Verification items for the finished model (mm, model axes). A direction names the side the tool comes from. Round coordinates to 2 decimals unless told otherwise and drop trailing zeros. Write each loop counter-clockwise with the first axis right and the second up, starting at its lowest first coordinate (ties: lowest second). Pieces come first, ordered by that corner, then holes. Notation, with made-up numbers: M 81.25,-1.75 L 89.25,-1.75 A36 cw 89.25,35.25 Z; hole C 3,-17 d4. An arc over 180 degrees is marked long. One line per question, with ' | ' between items.
from build123d import *

# Parameters (mm, degrees)
F0_W     = 278.8
F0_H     = 12.5
F4_DEPTH = 4
F6_D     = 8
F6_DEPTH = 25
F6_TIP   = 2.4034424761
F8_DEPTH = 4


with BuildPart() as f1:
    # F0 (on Front) → F1 (revolve)
    with BuildSketch(Plane.XZ):
        with Locations((139.4, 6.25)):
            Rectangle(F0_W, F0_H)
    revolve(axis=Axis((139.4, 0, 0), (-1, 0, 0)))

    # F3 (on offset) → F4 (cut)
    with BuildSketch(Plane.XY.offset(12.5)):
        with BuildLine():
            Line((0, 4), (0, 0))
            Line((0, 0), (0, -4))
            Line((0, -4), (108, -4))
            ThreePointArc((108, -4), (110.8284271247, -2.8284271247), (112, 0))
            ThreePointArc((112, 0), (110.8284271247, 2.8284271247), (108, 4))
            Line((108, 4), (0, 4))
        make_face()
    extrude(amount=-F4_DEPTH, mode=Mode.SUBTRACT)

    # F6
    with Locations(Plane(origin=(0, 0, 0), x_dir=(0, -1, 0), z_dir=(-1, 0, 0))):
        with Locations((0, 0)):
            Hole(F6_D / 2, depth=F6_DEPTH)
            with Locations((0, 0, -(F6_DEPTH + F6_TIP / 2))):  # 118° drill point
                Cone(0, F6_D / 2, F6_TIP, mode=Mode.SUBTRACT)

    # F7 (on offset) → F8 (cut)
    with BuildSketch(Plane.XY.offset(12.5)):
        with BuildLine():
            ThreePointArc((210.5, 0), (209.3284271247, 2.8284271247), (206.5, 4))
            Line((206.5, 4), (164.5, 4))
            ThreePointArc((164.5, 4), (161.6715728753, 2.8284271247), (160.5, 0))
            ThreePointArc((160.5, 0), (161.6715728753, -2.8284271247), (164.5, -4))
            Line((164.5, -4), (206.5, -4))
            ThreePointArc((206.5, -4), (209.3284271247, -2.8284271247), (210.5, 0))
        make_face()
    extrude(amount=-F8_DEPTH, mode=Mode.SUBTRACT)


solid = f1.part
1. Section check A-A, the plane y = 7.5. Record the cut outline in (x, z), then the cut area to 3 significant figures.
Results:
outline: M 0,-10 L 278.8,-10 L 278.8,10 L 0,10 Z | area: 5,580 mm2
2. Go/stop test with flat-tipped pins: P1, Ø2.5, axis at x = 182.5, z = 10, coming from the -Y side; P2, Ø2, axis at x = 138, z = 4.5, coming from the -Y side; P3, Ø4, axis at x = 107, z = 9.5, coming from the +Y side. Record where each tip stops, or that it passes through.
Results:
P1: stops at y = -8.93 | P2: stops at y = -12 | P3: stops at y = 10
3. Mould release check, pull along X, two halves, no side actions. Record for faces 3 (the face through (0, 3, -3)), 4 (the face through (141.352, -7.606, -9.92)), 5 (the face through (185, 0, 8.5)), 6 (the face through (278.8, 0, 0)): pulls with the +X half, pulls with the -X half, needs draft (parallel to the pull), parting line crosses it, or undercut.
Results:
face 3: pulls with the -X half | face 4: needs draft | face 5: undercut | face 6: pulls with the +X half
4. Thickness scan on line 1 (Y direction, x = 9, z = 0); line 2 (Y direction, x = 152, z = -1); line 3 (X direction, y = -1.25, z = 8.75). Record the ranges inside material, lowest first.
Results:
line 1: y = -12.5 to -4, 4 to 12.5 | line 2: y = -12.46 to 12.46 | line 3: x = 111.8 to 160.7, 210.3 to 278.8
5. Section check B-B, the plane y = -10.25. Record the cut outline in (x, z), then the cut area to 3 significant figures.
Results:
outline: M 0,-7.15 L 278.8,-7.15 L 278.8,7.15 L 0,7.15 Z | area: 3,990 mm2
6. Tool access check on faces 1 (the face through (55, 0, 8.5)), 2 (the face through (12.675, -0.867, -3.905)). Record the directions out of +Z, -Z, +X, -X, +Y, -Y that give a thin tool (end or side, any length) a straight path to the whole face; none if there is none.
Results:
face 1: +Z, -X | face 2: -X
